The listing builds one solid part. Answer for the finished solid, in the listing's coordinates (mm). A direction names the side the tool comes from. Give positions to 0.01 mm unless a question says otherwise; leave off trailing zeros. Write each loop counter-clockwise with the first axis right and the second up, starting at its lowest first coordinate (ties: lowest second). Pieces come first, ordered by that corner, then holes. Notation, with made-up numbers: (-8.5, 57) - (33.5, 57) arc R11 cw to (33.5, 66) - close; hole circle Ø5 at (3, -30). An arc over 180 degrees is marked (long way). Answer as CSV lines item,"result". Start each with the question number.
(1) Straight lines are drawn through the part: probe 1 along X at (y, z) = (190.5, -48.8) (3 decimals); probe 2 along Y at (x, z) = (48.65, -25.4) (3 decimals); probe 3 along X at (y, z) = (190, -49). For each, find the intervals that lie inside material, in ascending order.
(2) Find section C-C (z = -8). Write down the section's boundary in (x, y) (3 decimals).
(3) For a pull along X with two mould halves and no side action, classify faces 1 (the face through (50.8, 100, -25)), 2 (the face through (25, 100, -3.175)), 3 (the face through (49.235, 16.233, -26.865)), 4 (the face through (11.2, 9.9, -49.2)) as pulls with the +X half, pulls with the -X half, needs draft (parallel to the pull), parting line crosses it, or undercut.
(4) Each of these flat-tipped pins is pushed along its axis until it touches: pin 1 Ø4 at (y, z) = (184.15, -25.4) entering from -X; pin 2 Ø4 at (x, y) = (12.7, 190.5) entering from -Z (3 decimals); pin 3 Ø4 at (x, z) = (44.5, -7.5) entering from +Y. Where does it stop, or does it pass through?
(5) For faces 5 (the face through (3, 203.2, -26)), 6 (the face through (13.11, 193.65, -49.23)), 7 (the face through (49.235, 181.333, -26.865)), 8 (the face through (47.625, 100, -25)), determine the directions among +Z, -Z, +X, -X, +Y, -Y from which every point of the face is accessible in a straight line to the end or side of a thin tool.
(6) Find section B-B (y = 173). Write down the section's boundary in (x, z) (3 decimals), then the cut area to 3 significant figures.
(7) Find section A-A (x = 40). Write down the section's boundary in (y, z) (3 decimals).
(8) Find section D-D (x = 31.75). Write down the section's boundary in (y, z) (3 decimals), then the cut area to 3 significant figures.
from build123d import *

# Parameters (mm, degrees)
SKETCH1_W           = 50.8
SKETCH1_H           = 50.8
SKETCH1_W_2         = 44.45
SKETCH1_H_2         = 44.45
BOSS_EXTRUDE1_DEPTH = 203.2
SKETCH2_R           = 3.175
CUT_EXTRUDE1_DEPTH  = 24.638
SKETCH3_R           = 3.175
CUT_EXTRUDE2_DEPTH  = 24.638


with BuildPart() as part:
    # Sketch1 → Boss-Extrude1 (new body)
    with BuildSketch(Plane(origin=(0, 0, 0), x_dir=(1, 0, 0), z_dir=(0, 1, 0))):
        with Locations((25.4, 25.4)):
            Rectangle(SKETCH1_W, SKETCH1_H)
        with Locations((25.4, 25.4)):
            Rectangle(SKETCH1_W_2, SKETCH1_H_2, mode=Mode.SUBTRACT)
    extrude(amount=BOSS_EXTRUDE1_DEPTH)

    # Sketch2 → Cut-Extrude1 (cut)
    with BuildSketch(Plane(origin=(0, 0, -50.8), x_dir=(-1, 0, 0), z_dir=(0, 0, -1))):
        with Locations((-12.7, 190.5)):
            Circle(SKETCH2_R)
        with Locations((-31.75, 190.5)):
            Circle(SKETCH2_R)
        with Locations((-31.75, 12.7)):
            Circle(SKETCH2_R)
        with Locations((-12.7, 12.7)):
            Circle(SKETCH2_R)
    extrude(amount=-CUT_EXTRUDE1_DEPTH, mode=Mode.SUBTRACT)

    # Sketch3 → Cut-Extrude2 (cut)
    with BuildSketch(Plane(origin=(50.8, 0, 0), x_dir=(0, 0, -1), z_dir=(1, 0, 0))):
        with Locations((25.4, 184.15)):
            Circle(SKETCH3_R)
        with Locations((25.4, 19.05)):
            Circle(SKETCH3_R)
    extrude(amount=-CUT_EXTRUDE2_DEPTH, mode=Mode.SUBTRACT)


solid = part.part
Result set:
1,probe 1,"0 to 9.525, 15.875 to 28.575, 34.925 to 50.8"
1,probe 2,"0 to 15.875, 22.225 to 180.975, 187.325 to 203.2"
1,probe 3,"0 to 9.56, 15.84 to 28.61, 34.89 to 50.8"
2,outline,"(0, 0) - (3.175, 0) - (3.175, 203.2) - (0, 203.2) - close; (47.625, 0) - (50.8, 0) - (50.8, 203.2) - (47.625, 203.2) - close"
3,face 1,"pulls with the +X half"
3,face 2,"undercut"
3,face 3,"needs draft"
3,face 4,"undercut"
4,pin 1,"x = 0"
4,pin 2,"z = -3.175"
4,pin 3,"through"
5,face 5,"+Z, -Z, +X, -X, +Y"
5,face 6,"-Z"
5,face 7,"+X"
5,face 8,"+Y, -Y"
6,outline,"(0, -50.8) - (50.8, -50.8) - (50.8, 0) - (0, 0) - close; hole (3.175, -47.625) - (47.625, -47.625) - (47.625, -3.175) - (3.175, -3.175) - close"
6,area,"605 mm^2"
7,outline,"(0, -50.8) - (203.2, -50.8) - (203.2, -47.625) - (0, -47.625) - close; (0, -3.175) - (203.2, -3.175) - (203.2, 0) - (0, 0) - close"
8,outline,"(0, -50.8) - (9.525, -50.8) - (9.525, -47.625) - (0, -47.625) - close; (0, -3.175) - (203.2, -3.175) - (203.2, 0) - (0, 0) - close; (15.875, -50.8) - (187.325, -50.8) - (187.325, -47.625) - (15.875, -47.625) - close; (193.675, -50.8) - (203.2, -50.8) - (203.2, -47.625) - (193.675, -47.625) - close"
8,area,"1,250 mm^2"
